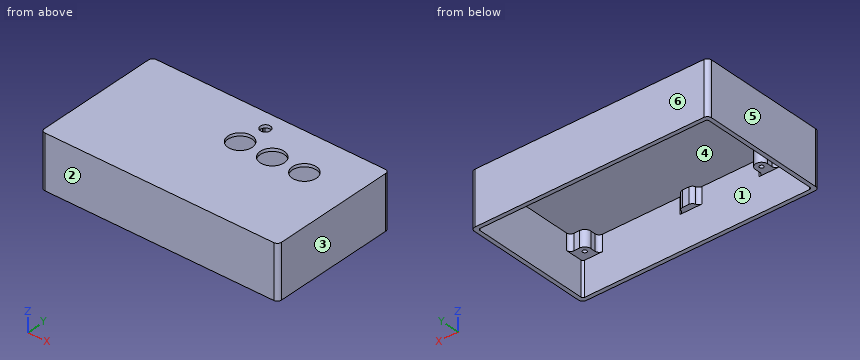
```python
from build123d import *

# Parameters (mm, degrees)
SKETCH2_W           = 118
SKETCH2_H           = 65
BOSS_EXTRUDE2_DEPTH = 1.5
SKETCH4_W           = 118
SKETCH4_H           = 65
SKETCH4_W_2         = 114
SKETCH4_H_2         = 61
BOSS_EXTRUDE3_DEPTH = 25
FILLET2_R           = 2
FILLET3_R           = 1
SKETCH5_R           = 6
SKETCH5_R_2         = 2.5
CUT_EXTRUDE1_DEPTH  = 27.5
SKETCH6_R           = 1
SKETCH6_W           = 7
SKETCH6_H           = 3
BOSS_EXTRUDE4_DEPTH = 8
FILLET4_R           = 2
FILLET6_R           = 2


with BuildPart() as part:
    # Sketch2 → Boss-Extrude2 (new body)
    with BuildSketch(Plane.XY):
        Rectangle(SKETCH2_W, SKETCH2_H)
    extrude(amount=BOSS_EXTRUDE2_DEPTH)

    # Sketch4 → Boss-Extrude3 (add)
    with BuildSketch(Plane.XY):
        Rectangle(SKETCH4_W, SKETCH4_H)
        Rectangle(SKETCH4_W_2, SKETCH4_H_2, mode=Mode.SUBTRACT)
    extrude(amount=-BOSS_EXTRUDE3_DEPTH)

    # Fillet2
    fillet2_edges = [part.edges().sort_by_distance(p)[0] for p in [
        (59, 32.5, -11.75),
        (59, -32.5, -11.75),
        (-59, -32.5, -11.75),
        (-59, 32.5, -11.75),
    ]]
    fillet(fillet2_edges, radius=FILLET2_R)

    # Fillet3
    fillet3_edges = [part.edges().sort_by_distance(p)[0] for p in [
        (-57, -30.5, -12.5),
        (-57, 30.5, -12.5),
        (57, 30.5, -12.5),
        (57, -30.5, -12.5),
    ]]
    fillet(fillet3_edges, radius=FILLET3_R)

    # Sketch5 → Cut-Extrude1 (cut, through all)
    with BuildSketch(Plane.XY.offset(1.5)):
        with Locations((35.125, 11)):
            Circle(SKETCH5_R)
        with Locations((19.125, 11)):
            Circle(SKETCH5_R)
        with Locations((3.125, 11)):
            Circle(SKETCH5_R)
        with Locations((4.625, 24)):
            Circle(SKETCH5_R_2)
    extrude(amount=-CUT_EXTRUDE1_DEPTH, mode=Mode.SUBTRACT)

    # Sketch6 → Boss-Extrude4 (add)
    with BuildSketch(Plane(origin=(0, 0, 0), x_dir=(-1, 0, 0), z_dir=(0, 0, -1))):
        with BuildLine():
            Line((-57, 30.5), (-57, 23))
            Line((-57, 23), (-52.125, 23))
            ThreePointArc((-52.125, 23), (-50.003679656, 23.878679656), (-49.125, 26))
            Line((-49.125, 26), (-49.125, 30.5))
            Line((-49.125, 30.5), (-57, 30.5))
        make_face()
        with Locations((-52.125, 26)):
            Circle(SKETCH6_R, mode=Mode.SUBTRACT)
        with BuildLine():
            Line((32.875, 30.5), (38.875, 30.5))
            Line((38.875, 30.5), (38.875, 26))
            ThreePointArc((38.875, 26), (35.875, 23), (32.875, 26))
            Line((32.875, 26), (32.875, 30.5))
        make_face()
        with Locations((35.875, 26)):
            Circle(SKETCH6_R, mode=Mode.SUBTRACT)
        with Locations((-3.125, 29)):
            Rectangle(SKETCH6_W, SKETCH6_H)
    boss_extrude4 = extrude(amount=BOSS_EXTRUDE4_DEPTH)

    # Mirror1: Boss-Extrude4 across plane
    add(boss_extrude4.mirror(Plane.ZX))

    # Fillet4
    fillet4_edges = [part.edges().sort_by_distance(p)[0] for p in [
        (49.125, 30.5, -4),
        (57, 23, -4),
        (-32.875, 30.5, -4),
        (-38.875, 30.5, -4),
        (-0.375, 30.5, -4),
        (6.625, 30.5, -4),
        (57, -23, -4),
        (49.125, -30.5, -4),
        (-32.875, -30.5, -4),
        (-38.875, -30.5, -4),
        (-0.375, -30.5, -4),
        (6.625, -30.5, -4),
    ]]
    fillet(fillet4_edges, radius=FILLET4_R)

    # Fillet6
    fillet6_edges = [part.edges().sort_by_distance(p)[0] for p in [
        (-0.375, 27.5, -4),
        (6.625, 27.5, -4),
        (6.625, -27.5, -4),
        (-0.375, -27.5, -4),
    ]]
    fillet(fillet6_edges, radius=FILLET6_R)


solid = part.part
```
Here's how the part is built. I have some questions about the finished solid (model axes, mm). Face numbers are marked on the shaded views. A direction names the side the tool comes from. Give positions to 0.01 mm unless a question says otherwise; leave off trailing zeros. Order: outer loops, then holes, each group sorted by start corner. A loop starts at its lowest first (then second) coordinate and runs counter-clockwise, first axis right, second up. Notation, with made-up numbers: M 28.25,13 L 69.25,13 A28 ccw 69.25,32 Z; hole C -39.5,56 d2. An arc over 180 degrees is marked long. Use a Markdown table: item, result. Add a question column.
1. For pin 1 Ø2 at (x, y) = (-35.5, 26.5) entering from -Z; pin 2 Ø1.2 at (x, y) = (-35.875, 26) entering from -Z, each with a flat end and sliding along its axis, tell me the tip position at first contact or that it passes through.
2. If we mould it in two halves opening along X, with no side actions, what happens to the marked faces 3, 4, 5 and 6? For each: +X half, -X half, draft (parallel to the pull), parting line (faces both ways), or undercut.
3. Suppose I cut it at A-A (y = 11). List the corners of the cut face in (x, z) for me (3 decimals), and give its area (3 significant figures).
4. Suppose I cut it at D-D (z = -3.75). Give the number of separate pieces and of enclosed holes in the cut face, and give its area (3 significant figures).
5. On a 3-axis mill with a long thin cutter (end or side, diameter ignored), from which of +Z, -Z, +X, -X, +Y, -Y can I reach the whole of each face in a straight line? I mean the marked faces 1 and 2. Say none if no direction works.
6. I need wall thicknesses on probe 1 along X at (y, z) = (-26, -5) (3 decimals); probe 2 along Y at (x, z) = (21, -13.75); probe 3 along X at (y, z) = (-11, -6). Which ranges of each line are inside material? Lowest first, please. Write a range as from..to.
7. Suppose I cut it at C-C (y = -12.5). List the corners of the cut face in (x, z) for me, and give its area (3 significant figures).
8. Suppose I cut it at B-B (x = -21.5). List the corners of the cut face in (y, z) for me, and give its area (4 significant figures).
Results list:
| question | item | result |
|---|---|---|
| 1 | pin 1 | stops at z = -8 |
| 1 | pin 2 | stops at z = 0 |
| 2 | face 3 | +X half |
| 2 | face 4 | undercut |
| 2 | face 5 | -X half |
| 2 | face 6 | draft |
| 3 | outline | M -59,-25 L -57,-25 L -57,0 L -2.875,0 L -2.875,1.5 L -59,1.5 Z; M 9.125,0 L 13.125,0 L 13.125,1.5 L 9.125,1.5 Z; M 25.125,0 L 29.125,0 L 29.125,1.5 L 25.125,1.5 Z; M 41.125,0 L 57,0 L 57,-25 L 59,-25 L 59,1.5 L 41.125,1.5 Z |
| 3 | area | 223 mm² |
| 4 | separate pieces | 1 |
| 4 | enclosed holes | 5 |
| 4 | area | 947 mm² |
| 5 | face 1 | -Z |
| 5 | face 2 | +Z, -Z, +X, -X, -Y |
| 6 | probe 1 | x = -59..-57, -38.875..-36.875, -34.875..-32.875, 49.125..51.125, 53.125..59 |
| 6 | probe 2 | y = -32.5..-30.5, 30.5..32.5 |
| 6 | probe 3 | x = -59..-57, 57..59 |
| 7 | outline | M -59,-25 L -57,-25 L -57,0 L 57,0 L 57,-25 L 59,-25 L 59,1.5 L -59,1.5 Z |
| 7 | area | 277 mm² |
| 8 | outline | M -32.5,-25 L -30.5,-25 L -30.5,0 L 30.5,0 L 30.5,-25 L 32.5,-25 L 32.5,1.5 L -32.5,1.5 Z |
| 8 | area | 197.5 mm² |
